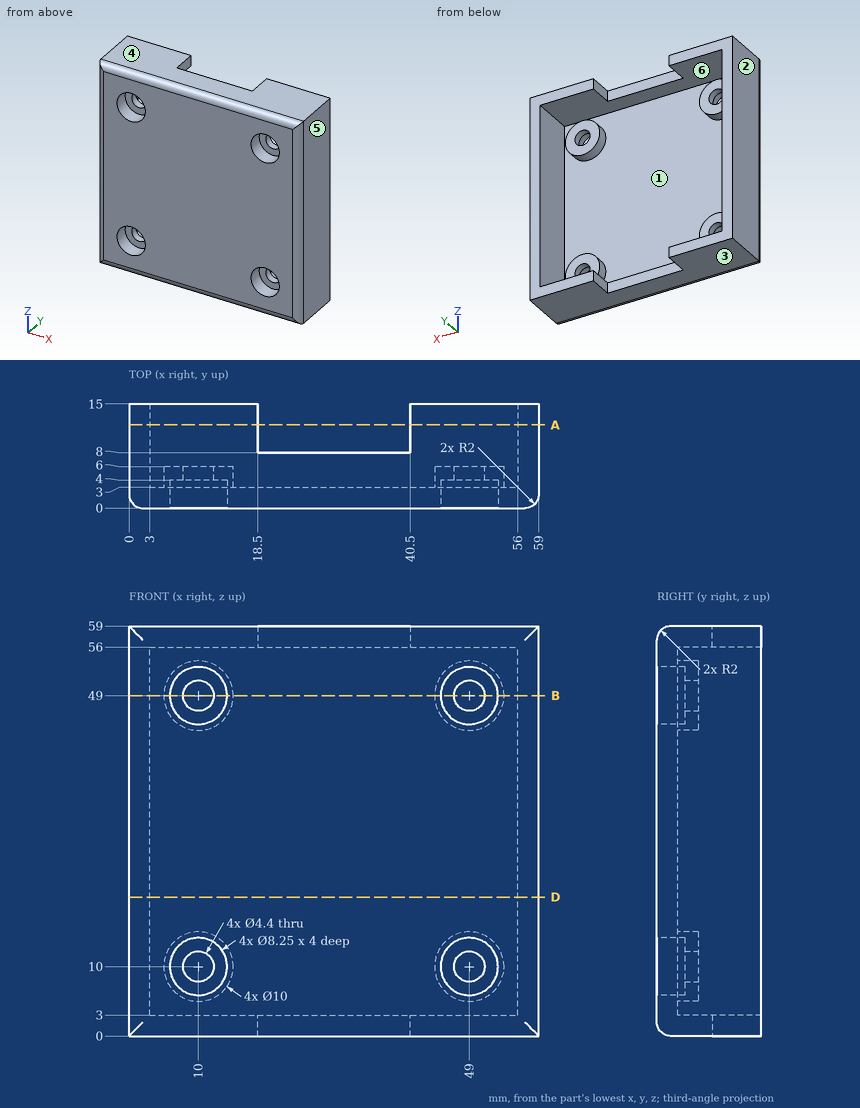
Study the drawing (mm; zero at the part's minimum x, y, z) and answer. A direction names the side the tool comes from. Round coordinates to 2 decimals unless told otherwise and drop trailing zeros. Write each loop counter-clockwise with the first axis right and the second up, starting at its lowest first coordinate (ties: lowest second). Pieces come first, ordered by that corner, then holes.
1) A cutting plane is placed at D-D (z = 20). Give the vertices of the cut face in (x, y), plus the area to 3 significant figures.
2) A cutting plane is placed at A-A (y = 12). Give the vertices of the cut face in (x, z).
3) Straight lines are drawn through the part: line 1 (Z direction, x = 10, y = 4.7); line 2 (Z direction, x = 10, y = 2.9) (3 decimals); line 3 (X direction, y = 9, z = 5.5). For each, find the intervals that lie inside material, in ascending order.
4) The mould has two halves that part along Z. Classify the marked faces 3, 4, 5 and 6: pulls with the +Z half, pulls with the -Z half, needs draft (parallel to the pull), parting line crosses it, or undercut.
5) A cutting plane is placed at B-B (z = 49). Give the number of separate pieces and of enclosed holes in the cut face, plus the area to 3 significant figures.
6) A tool of negligible diameter and unlimited length cuts with its end or side. For the marked faces 1 and 2, from which of +Z, -Z, +X, -X, +Y, -Y can it reach the whole face along a straight path? Write none if from no direction.
7) Given pin 1 Ø3 at (x, z) = (47.5, 12.5) entering from +Y; pin 2 Ø7 at (x, z) = (49, 49) entering from -Y; pin 3 Ø1.5 at (x, z) = (32, 58) entering from +Y, each flat-ended and moving along its own axis, determine where each tip first touches the part or whether it passes through.
Completed:
1. outline: (0, 2) arc R2 ccw to (2, 0) - (57, 0) arc R2 ccw to (59, 2) - (59, 15) - (56, 15) - (56, 3) - (3, 3) - (3, 15) - (0, 15) - close
1. area: 247 mm2
2. outline: (0, 0) - (18.5, 0) - (18.5, 3) - (3, 3) - (3, 56) - (18.5, 56) - (18.5, 59) - (0, 59) - close; (40.5, 0) - (59, 0) - (59, 59) - (40.5, 59) - (40.5, 56) - (56, 56) - (56, 3) - (40.5, 3) - close
3. line 1: z = 0 to 3, 5 to 7.8, 12.2 to 15, 44 to 46.8, 51.2 to 54, 56 to 59
3. line 2: z = 0 to 5.875, 14.125 to 44.875, 53.125 to 59
3. line 3: x = 0 to 3, 56 to 59
4. face 3: pulls with the -Z half
4. face 4: pulls with the +Z half
4. face 5: needs draft
4. face 6: undercut
5. separate pieces: 3
5. enclosed holes: 0
5. area: 224 mm2
6. face 1: +Y
6. face 2: +Z, -Z, -X, +Y, -Y
7. pin 1: stops at y = 6
7. pin 2: stops at y = 4
7. pin 3: stops at y = 8
